Autodesk Inventor part; units mm, degrees
ref_plane "YZ Plane" through (0, 0, 0) normal (1, 0, 0) x (0, 1, 0)
ref_plane "XZ Plane" through (0, 0, 0) normal (0, 1, 0) x (-1, 0, 0)
ref_plane "XY Plane" through (0, 0, 0) normal (0, 0, 1) x (1, 0, 0)
sketch "Sketch1" plane through (0, 0, 0) normal (0, 0, 1) x (1, 0, 0)
  line L0 (-85.3474, 52.3284) -> (-82.8074, 52.3284)
  line L1 (-82.8074, 52.3284) -> (-82.8074, 7.8784)
  line L2 (-82.8074, 7.8784) -> (-85.3474, 7.8784)
  line L3 (-85.3474, 7.8784) -> (-85.3474, 52.3284)
  point P0 (0, 0)
  dimension "d0" = 2.54
  dimension "d1" = 44.45
revolve "Revolution1" add sketch "Sketch1" angle 360 about axis through (-85.3474, 7.8784, 0) along (0, 1, 0)
sketch "Sketch2" plane through (-85.3474, 52.3284, 0) normal (0, 1, 0) x (1, 0, 0)
  circle A0 centre (0, 0) radius 2.54
  line L0 (6.1828, 0) -> (3.0914, -5.3544)
  line L1 (3.0914, -5.3544) -> (-3.0914, -5.3544)
  line L2 (-3.0914, -5.3544) -> (-6.1828, 0)
  line L3 (-6.1828, 0) -> (-3.0914, 5.3544)
  line L4 (-3.0914, 5.3544) -> (3.0914, 5.3544)
  line L5 (3.0914, 5.3544) -> (6.1828, 0)
  point P0 (85.3474, 0)
extrude "Extrusion1" add sketch "Sketch2" along normal blind 3.81 contours A0 | L0 L1 L2 L3 L4 L5
sketch "Sketch3" plane through (-85.3474, 56.1384, 0) normal (0, 1, 0) x (1, 0, 0)
  line L0 (-3.0914, 5.3544) -> (3.0914, 5.3544)
  ellipse E0 centre (0, 1.4435) end of major axis (0, 0.4462) minor radius 1.8269
  spline S0 degree 5 poles (-0.9642, 1.0834) (-0.9417, 0.9678) (-0.7135, 0.7937) (0.1443, 0.7781) (1.4903, 0.7931) (0.5526, 1.6401) (0.1051, 0.6276) (-0.4914, 1.4752) (-0.8935, 1.3263) (-0.9814, 1.1718) (-0.9642, 1.0834) knots 0 0 0 0 0 0 0.230424 0.370543 0.547944 0.706233 0.823711 1 1 1 1 1 1
  circle A0 centre (-0.9642, 1.8591) radius 0.1959
  circle A1 centre (0.6426, 1.8591) radius 0.277
  point P0 (85.3474, 0)
  point P1 (0.9196, 1.0834)
  point P2 (0.6426, 1.2496)
  point P3 (0, 1.0834)
  point P4 (-0.7703, 1.305)
extrude "Extrusion2" cut sketch "Sketch3" against normal blind 0.508
properties part number ".2'' diameter 2.5 inch bolts for wheel"
The listing builds one solid part. Answer for the finished solid, in the listing's coordinates (mm). A direction names the side the tool comes from. Give positions to 0.01 mm unless a question says otherwise; leave off trailing zeros. Order: outer loops, then holes, each group sorted by start corner. A loop starts at its lowest first (then second) coordinate and runs counter-clockwise, first axis right, second up. Notation, with made-up numbers: (40, 5.5) -> (83, 5.5) arc R13 ccw to (83, 30.5) -> close; hole circle Ø7 at (59, 86.5). An arc over 180 degrees is marked (long way). Write each question's results on one line, items separated by ' | '.
Q1. The part is cut by section B-B, the plane x = -89. Give the vertices of the cut face in (y, z).
Checked values:
outline: (52.33, -4.38) -> (56.14, -4.38) -> (56.14, 4.38) -> (52.33, 4.38) -> close
Q2. Which of the six approach directions +Z, -Z, +X, -X, +Y, -Y give full straight-line access (tool end or side, diameter ignored) to faces 1 (the face through (-85, 56.138, 0)), 2 (the face through (-83, 29.79, -0.97))?
Checked values:
face 1: +Z, -Z, +X, -X, +Y | face 2: -Y
Q3. Straight lines are drawn through the part: probe 1 along Y at (x, z) = (-82.5, 5); probe 2 along Z at (x, y) = (-85.25, 16); probe 3 along X at (y, z) = (48, -1). For each, find the intervals that lie inside material, in ascending order. Write a range as from..to.
Checked values:
probe 1: y = 52.33..56.14 | probe 2: z = -2.54..2.54 | probe 3: x = -87.68..-83.01
Q4. Determine the mould class of faces 3 (the face through (-89.963, 54.207, 2.715)), 4 (the face through (-85.4, 55.63, -1.5)), 5 (the face through (-85, 54, -5.354)), 6 (the face through (-85, 7.878, 0)) for opening direction Z: pulls with the +Z half, pulls with the -Z half, needs draft (parallel to the pull), parting line crosses it, or undercut.
Checked values:
face 3: pulls with the +Z half | face 4: undercut | face 5: pulls with the -Z half | face 6: needs draft
Q5. Each of these flat-tipped pins is pushed along its axis until it touches: P1, Ø6, axis at y = 13.5, z = 3, coming from the +X side; P2, Ø6, axis at x = -90, y = 35.5, coming from the +Z side; P3, Ø1, axis at x = -87, y = 13, coming from the -Z side. Where does it stop, or does it pass through?
Checked values:
P1: stops at x = -82.81 | P2: stops at z = 1.93 | P3: stops at z = -2.26
Q6. The part is cut by section A-A, the plane y = 26. Give the vertices of the cut face in (x, z), and give its area (3 significant figures).
Checked values:
outline: circle Ø5.08 at (-85.35, 0) | area: 20.3 mm^2
